Verification items for the finished model (mm, model axes). A direction names the side the tool comes from. Give positions to 0.01 mm unless a question says otherwise; leave off trailing zeros. Order: outer loops, then holes, each group sorted by start corner. A loop starts at its lowest first (then second) coordinate and runs counter-clockwise, first axis right, second up. Notation, with made-up numbers: (32, 81.25) -> (74, 81.25) arc R7 ccw to (74, 91.25) -> close; hole circle Ø11 at (-12.5, 55). An arc over 180 degrees is marked (long way). Write each question's results on one line, items separated by ' | '. Start each with the question number.
1. Cross-section at B-B, the plane x = -6.25. Enter the section's corners in (y, z), then the cut area to 3 significant figures.
2. Material ranges on L1, parallel to Z at x = 0, y = -17.45; L2, parallel to X at y = -12, z = -1; L3, parallel to Y at x = 9.75, z = -5.5, recorded low to high. Write a range as from..to.
3. Cross-section at A-A, the plane y = -18. Enter the section's corners in (x, z), then the cut area to 3 significant figures.
4. Set-up check for faces 5 (the face through (0, -16.202, -6)), 6 (the face through (0, -13.736, -6)), 7 (the face through (-5, -10.49, -6)), 8 (the face through (7, -12.7, -6)), 9 (the face through (-3.876, -13, -6)): record each of +Z, -Z, +X, -X, +Y, -Y from which the full face is reachable in a straight line by a thin tool's end or side.
5. Mould release check, pull along X, two halves, no side actions. Record for faces 1 (the face through (1.218, -11, -6)), 2 (the face through (5, -10.49, -6)), 3 (the face through (-9.55, -16, -6)), 4 (the face through (-2.7, -7.7, -6.3)): +X half, -X half, draft (parallel to the pull), parting line (faces both ways), or undercut.
6. Cross-section at C-C, the plane x = 0. Enter the section's corners in (y, z).
7. Depth check by flat-ended pin: pin 1 Ø1.9 at (x, z) = (0, -5) entering from +Y; pin 2 Ø1.9 at (x, z) = (7, -7) entering from +Y; pin 3 Ø2.5 at (y, z) = (-11, -3.5) entering from -X. Enter the tip coordinate at first touch or a pass-through.
from build123d import *

# Parameters (mm, degrees)
BOSS_EXTRUDE1_DEPTH = 12.7
SKETCH10_R          = 3.082136138
CUT_EXTRUDE1_DEPTH  = 26.185474767
SKETCH11_W          = 2.435876878
SKETCH11_H          = 7.908405343
CUT_EXTRUDE2_DEPTH  = 26.185474767
FILLET1_R           = 0.635
FILLET3_R           = 0.508
SKETCH17_W          = 0.605016918
SKETCH17_H          = 2.095446093
SKETCH17_W_2        = 0.604461085
SKETCH17_H_2        = 2.141007526
CUT_EXTRUDE7_DEPTH  = 26.185474767
SKETCH18_R          = 5.08
CUT_EXTRUDE8_DEPTH  = 2.794


with BuildPart() as part:
    # Sketch5 → Boss-Extrude1 (new body)
    with BuildSketch(Plane.XY):
        Polygon((-6.474794456, -10.4902), (-6.938297275, -10.378313453), (-7.308763147, -10.05450356), (-7.490794456, -9.4742), (-7.378907909, -9.01069718), (-7.193214945, -8.75577951), (-3.863171405, -5.42573597), (-2.833127272, -4.737482484), (-1.618107374, -4.4958), (1.618107374, -4.4958), (2.668236067, -4.674493152), (3.863171405, -5.42573597), (7.193214945, -8.75577951), (7.490794456, -9.4742), (7.378907909, -9.93770282), (6.938297275, -10.378313453), (6.474794456, -10.4902), (4.3434, -10.4902), (3.646537163, -10.737670005), (3.377082754, -11.059343535), (3.2385, -11.5951), (3.485970005, -12.291962837), (3.807643535, -12.561417246), (4.3434, -12.7), (10.5918, -12.7), (10.5918, -18.995576116), (-9.5504, -18.995576116), (-9.5504, -12.7), (-4.3434, -12.7), (-3.863171405, -12.590180165), (-3.485969976, -12.291962837), (-3.271081829, -11.861441531), (-3.271081829, -11.328758469), (-3.485969976, -10.898237163), (-3.863171405, -10.600019835), (-4.3434, -10.4902), align=None)
    extrude(amount=-BOSS_EXTRUDE1_DEPTH)

    # Sketch10 → Cut-Extrude1 (cut, through all)
    with BuildSketch(Plane.XY):
        with Locations((-0.066530556, -6.095976424)):
            Circle(SKETCH10_R)
    extrude(amount=-CUT_EXTRUDE1_DEPTH, mode=Mode.SUBTRACT)

    # Sketch11 → Cut-Extrude2 (cut, through all)
    with BuildSketch(Plane.XY):
        with Locations((0, -9.781904855)):
            Rectangle(SKETCH11_W, SKETCH11_H)
    extrude(amount=-CUT_EXTRUDE2_DEPTH, mode=Mode.SUBTRACT)

    # Fillet1
    fillet1_edges = [part.edges().sort_by_distance(p)[0] for p in [
        (-9.5504, -12.7, -6.35),
    ]]
    fillet(fillet1_edges, radius=FILLET1_R)

    # Fillet3
    # the kernel refuses this fillet: 0.508 mm, written as the material it takes off along each edge
    with BuildSketch(Plane(origin=(2.668236067, -4.674493152, 3.28944818), x_dir=(0.8465916632907232, -0.5322429479538895, 0), z_dir=(0, 0, -1))) as fillet3_piece_1:
        with BuildLine():
            CenterArc((1.315779272, 0.508), FILLET3_R, 143.192029884, 126.807970116)
            Line((0.90905007, 0.812360569), (0.900915486, 0.81844778))
            ThreePointArc((0.900915486, 0.81844778), (0.488321858, 0.368360866), (-0.005137978, 0.008765089))
            Line((-0.005137978, 0.008765089), (0, -0.01016))
            Line((0, -0.01016), (1.315779272, -0.01016))
            Line((1.315779272, -0.01016), (1.315779272, 0))
        make_face()
    extrude(amount=19.278896361, mode=Mode.SUBTRACT)
    with BuildSketch(Plane(origin=(-2.833127272, -4.737482484, 3.097058862), x_dir=(-0.8314696122997464, -0.5555702330237908, 0), z_dir=(0, 0, -1))) as fillet3_piece_2:
        with BuildLine():
            CenterArc((1.31839441, -0.501729486), FILLET3_R, 99.011665767, 118.073467257)
            Line((0.913142276, -0.808054001), (0.905037233, -0.814180491))
            ThreePointArc((0.905037233, -0.814180491), (0.490196501, -0.366028623), (-0.005094947, -0.008790172))
            Line((-0.005094947, -0.008790172), (0, 0.01016))
            ThreePointArc((0, 0.01016), (0.619411772, 0.01016), (1.237232128, 0.01003459))
            Line((1.237232128, 0.01003459), (1.238823545, 0))
        make_face()
    extrude(amount=18.894117724, mode=Mode.SUBTRACT)

    # Sketch17 → Cut-Extrude7 (cut, through all)
    with BuildSketch(Plane.XY):
        with Locations((3.55718824, -12.68838448)):
            Rectangle(SKETCH17_W, SKETCH17_H)
        with Locations((-3.573312372, -12.665603763)):
            Rectangle(SKETCH17_W_2, SKETCH17_H_2)
    extrude(amount=-CUT_EXTRUDE7_DEPTH, mode=Mode.SUBTRACT)

    # Sketch18 → Cut-Extrude8 (cut)
    with BuildSketch(Plane.XZ.offset(18.995576116)):
        with Locations((0, -6.35)):
            Circle(SKETCH18_R)
    extrude(amount=-CUT_EXTRUDE8_DEPTH, mode=Mode.SUBTRACT)


solid = part.part
Results below:
1) outline: (-19, -12.7) -> (-12.7, -12.7) -> (-12.7, 0) -> (-19, 0) -> close; (-10.49, -12.7) -> (-7.81, -12.7) -> (-7.81, 0) -> (-10.49, 0) -> close | area: 114 mm²
2) L1: z = -12.7..-11.43, -1.27..0 | L2: x = -3.27..-1.22, 1.22..3.25 | L3: y = -19..-12.7
3) outline: (-9.55, -12.7) -> (10.59, -12.7) -> (10.59, 0) -> (-9.55, 0) -> close; hole circle Ø10.16 at (0, -6.35) | area: 175 mm²
4) face 5: -Y | face 6: +Z, -Z, +Y | face 7: +Z, -Z, -X | face 8: +Z, -Z, +X | face 9: +Z, -Z
5) face 1: undercut | face 2: draft | face 3: -X half | face 4: undercut
6) outline: (-19, -12.7) -> (-13.74, -12.7) -> (-13.74, 0) -> (-19, 0) -> (-19, -1.27) -> (-16.2, -1.27) -> (-16.2, -11.43) -> (-19, -11.43) -> close
7) pin 1: stops at y = -13.74 | pin 2: stops at y = -7.61 | pin 3: stops at x = -7.4
